The model under review builds one solid part; all positions refer to its coordinate system, in mm. A direction names the side the tool comes from. Give positions to 0.01 mm unless a question says otherwise; leave off trailing zeros. Loops run counter-clockwise (first coordinate to the right, second up) from the corner with the lowest first, then second, coordinate; pieces in that order, holes last. Notation, with made-up numbers: (79, 21.5) -> (110, 21.5) arc R15 ccw to (110, 45.5) -> close; hole circle Ø3 at (23.25, 68). An arc over 180 degrees is marked (long way). Write each question's results on one line, items separated by ' | '. Start each with the question number.
Q1. We need section D-D (x = -20). Write out the cut boundary in (y, z).
Q2. We need section A-A (y = 18.5). Write out the cut boundary in (x, z), plus the area to 3 significant figures.
Q3. We need section C-C (y = 23.5). Write out the cut boundary in (x, z), plus the area to 3 significant figures.
Q4. Insertion check: pin 1 Ø10 at (x, y) = (-17, 24.5) entering from +Z; pin 2 Ø2 at (x, z) = (3, 13.5) entering from +Y; pin 3 Ø10 at (y, z) = (15.5, 11.5) entering from +X. Each pin has a flat end and moves straight along its axis. Give the tip position at first contact, or say it passes through.
Q5. Wall thickness on L1, parallel to Z at x = 6.5, y = 15.75; L2, parallel to Y at x = -5, z = 88; L3, parallel to Y at x = -25, z = 60: over which ranges is each line inside the solid? List them lowest first. Write a range as [from, to].
Q6. Machinability: for faces 5 (the face through (20, 6, 36)), 6 (the face through (-23, 1, 44.75)), 7 (the face through (-18, 21.5, 88)), 8 (the face through (24, 20, 12)), 9 (the face through (-17, 25, 81)), which of the approach directions +Z, -Z, +X, -X, +Y, -Y give a long, thin tool a straight path to every point of the face, cutting with its end or side? Answer none if there is none.
Q7. We need section B-B (z = 26). Write out the cut boundary in (x, y).
Q8. Mouldability with a two-part tool opening along Z and no side actions: class faces 1 (the face through (-29.116, 9.513, 1.141)), 2 (the face through (0, 8, 94)), 3 (the face through (-6, 15, 93)), 4 (the face through (-7, 15.5, 36)) as released by +Z, released by -Z, zero draft, split by the parting line, or undercut.
from build123d import *

# Parameters (mm, degrees)
BOSS_EXTRUDE1_DEPTH = 94
SKETCH2_W           = 14
SKETCH2_H           = 14
CUT_EXTRUDE1_DEPTH  = 5
SKETCH3_W           = 52
SKETCH3_H           = 12
BOSS_EXTRUDE2_DEPTH = 25
SKETCH4_W           = 6
SKETCH4_H           = 48
BOSS_EXTRUDE3_DEPTH = 10
SKETCH5_W           = 13.5
SKETCH5_H           = 11
SKETCH5_W_2         = 13
SKETCH5_H_2         = 6
CUT_EXTRUDE2_DEPTH  = 10
CUT_EXTRUDE3_DEPTH  = 2
SKETCH7_W           = 19
SKETCH7_H           = 2.5
CUT_EXTRUDE4_DEPTH  = 102.056914657
SKETCH8_R           = 4
CUT_EXTRUDE5_DEPTH  = 10
BOSS_EXTRUDE5_DEPTH = 2
FILLET2_R           = 4
FILLET3_R           = 4
SKETCH10_W          = 15
SKETCH10_H          = 15
BOSS_EXTRUDE6_DEPTH = 0.5


# Some blends are built 0.0001 mm under size
with BuildPart() as part:
    # Sketch1 → Boss-Extrude1 (new body)
    with BuildSketch(Plane.XY):
        with BuildLine():
            Line((-31.5, 15.5), (-28.5, 0))
            Line((-28.5, 0), (-21, 0))
            ThreePointArc((-21, 0), (0, 1.776625594), (21, 0))
            Line((21, 0), (28.5, 0))
            Line((28.5, 0), (31.5, 15.5))
            Line((31.5, 15.5), (-31.5, 15.5))
        make_face()
    extrude(amount=BOSS_EXTRUDE1_DEPTH)

    # Sketch2 → Cut-Extrude1 (cut)
    with BuildSketch(Plane(origin=(0, 0, 0), x_dir=(-1, 0, 0), z_dir=(0, 0, -1))):
        Rectangle(SKETCH2_W, SKETCH2_H)
    extrude(amount=-CUT_EXTRUDE1_DEPTH, mode=Mode.SUBTRACT)

    # Sketch3 → Boss-Extrude2 (add)
    with BuildSketch(Plane.XY.offset(94)):
        with Locations((0, 21.5)):
            Rectangle(SKETCH3_W, SKETCH3_H)
    extrude(amount=-BOSS_EXTRUDE2_DEPTH)

    # Sketch4 → Boss-Extrude3 (add)
    with BuildSketch(Plane(origin=(0, 15.5, 0), x_dir=(1, 0, 0), z_dir=(0, 1, 0))):
        with Locations((24, -36)):
            Rectangle(SKETCH4_W, SKETCH4_H)
    extrude(amount=BOSS_EXTRUDE3_DEPTH)

    # Sketch5 → Cut-Extrude2 (cut)
    with BuildSketch(Plane.XY.offset(94)):
        with Locations((-18.25, 16)):
            Rectangle(SKETCH5_W, SKETCH5_H)
        with Locations((1, 22.5)):
            Rectangle(SKETCH5_W_2, SKETCH5_H_2)
        with Locations((19, 22.5)):
            Rectangle(SKETCH5_W_2, SKETCH5_H_2)
        with Locations((1, 13)):
            Rectangle(SKETCH5_W_2, SKETCH5_H_2)
        with Locations((19, 13)):
            Rectangle(SKETCH5_W_2, SKETCH5_H_2)
    extrude(amount=-CUT_EXTRUDE2_DEPTH, mode=Mode.SUBTRACT)

    # Sketch6 → Cut-Extrude3 (cut)
    with BuildSketch(Plane.XY.offset(94)):
        Polygon((-26, 15.5), (-26, 9.5), (-10.5, 9.5), (-10.5, 19.5), (-6, 19.5), (-6, 9.5), (8, 9.5), (8, 19.5), (12, 19.5), (12, 9.5), (26, 9.5), (26, 33.954249065), (-26, 33.954249065), align=None)
    extrude(amount=-CUT_EXTRUDE3_DEPTH, mode=Mode.SUBTRACT)

    # Sketch7 → Cut-Extrude4 (cut, through all)
    with BuildSketch(Plane.XY.offset(92)):
        with Locations((-16.5, 26.25)):
            Rectangle(SKETCH7_W, SKETCH7_H)
    extrude(amount=-CUT_EXTRUDE4_DEPTH, mode=Mode.SUBTRACT)

    # Sketch8 → Cut-Extrude5 (cut)
    with BuildSketch(Plane.XZ):
        with BuildLine():
            ThreePointArc((-21, 57.872983346), (-23.16227766, 56.449489743), (-24, 54))
            ThreePointArc((-24, 54), (-23.16227766, 51.550510257), (-21, 50.127016654))
            Line((-21, 50.127016654), (-21, 57.872983346))
        make_face()
        with BuildLine():
            ThreePointArc((-16, 54), (-17.550510257, 57.16227766), (-21, 57.872983346))
            Line((-21, 57.872983346), (-21, 50.127016654))
            ThreePointArc((-21, 50.127016654), (-17.550510257, 50.83772234), (-16, 54))
        make_face()
        with BuildLine():
            ThreePointArc((-21, 43.872983346), (-23.16227766, 42.449489743), (-24, 40))
            ThreePointArc((-24, 40), (-23.16227766, 37.550510257), (-21, 36.127016654))
            Line((-21, 36.127016654), (-21, 43.872983346))
        make_face()
        with BuildLine():
            ThreePointArc((-16, 40), (-17.550510257, 43.16227766), (-21, 43.872983346))
            Line((-21, 43.872983346), (-21, 36.127016654))
            ThreePointArc((-21, 36.127016654), (-17.550510257, 36.83772234), (-16, 40))
        make_face()
        with BuildLine():
            ThreePointArc((-16, 54), (-17.550510257, 50.83772234), (-21, 50.127016654))
            Line((-21, 50.127016654), (-21, 43.872983346))
            ThreePointArc((-21, 43.872983346), (-17.550510257, 43.16227766), (-16, 40))
            Line((-16, 40), (-16, 54))
        make_face()
        with BuildLine():
            ThreePointArc((-21, 50.127016654), (-23.16227766, 51.550510257), (-24, 54))
            Line((-24, 54), (-24, 40))
            ThreePointArc((-24, 40), (-23.16227766, 42.449489743), (-21, 43.872983346))
            Line((-21, 43.872983346), (-21, 50.127016654))
        make_face()
        with Locations((20, 54)):
            Circle(SKETCH8_R)
        with BuildLine():
            Line((24, 40), (24, 54))
            ThreePointArc((24, 54), (20, 50), (16, 54))
            Line((16, 54), (16, 40))
            ThreePointArc((16, 40), (20, 44), (24, 40))
        make_face()
        with Locations((20, 40)):
            Circle(SKETCH8_R)
    extrude(amount=-CUT_EXTRUDE5_DEPTH, mode=Mode.SUBTRACT)

    # Sketch9 → Boss-Extrude5 (add)
    with BuildSketch(Plane.XZ):
        with BuildLine():
            Line((-15, 40), (-15, 54))
            ThreePointArc((-15, 54), (-16.83772234, 57.872983346), (-21, 58.898979486))
            Line((-21, 58.898979486), (-21, 57.872983346))
            ThreePointArc((-21, 57.872983346), (-17.550510257, 57.16227766), (-16, 54))
            Line((-16, 54), (-16, 44.75))
            Line((-16, 44.75), (-18.25, 44.75))
            Line((-18.25, 44.75), (-18.25, 40))
            ThreePointArc((-18.25, 40), (-20, 38.25), (-21.75, 40))
            Line((-21.75, 40), (-21.75, 44.75))
            Line((-21.75, 44.75), (-25, 44.75))
            Line((-25, 44.75), (-25, 40))
            ThreePointArc((-25, 40), (-20, 35), (-15, 40))
        make_face()
        with BuildLine():
            Line((16, 44.75), (18.25, 44.75))
            Line((18.25, 44.75), (18.25, 40))
            ThreePointArc((18.25, 40), (20, 38.25), (21.75, 40))
            Line((21.75, 40), (21.75, 44.75))
            Line((21.75, 44.75), (25, 44.75))
            Line((25, 44.75), (25, 40))
            ThreePointArc((25, 40), (20, 35), (15, 40))
            Line((15, 40), (15, 54))
            ThreePointArc((15, 54), (16.83772234, 57.872983346), (21, 58.898979486))
            Line((21, 58.898979486), (21, 57.872983346))
            ThreePointArc((21, 57.872983346), (17.550510257, 57.16227766), (16, 54))
            Line((16, 54), (16, 44.75))
        make_face()
    extrude(amount=-BOSS_EXTRUDE5_DEPTH)

    # Fillet2
    fillet2_edges = [part.edges().sort_by_distance(p)[0] for p in [
        (-28.5, 0, 47),
        (28.5, 0, 47),
    ]]
    fillet(fillet2_edges, radius=FILLET2_R)

    # Fillet3
    fillet3_edges = [part.edges().sort_by_distance(p)[0] for p in [
        (30.313539907, 9.369956187, 0),
        (27.745510401, 0.914521876, 0),
        (23.099980206, 0, 0),
    ]]
    fillet(fillet3_edges, radius=FILLET3_R)
    fillet3_2_edges = [part.edges().sort_by_distance(p)[0] for p in [
        (-30.313539907, 9.369956187, 0),
        (-27.745510401, 0.914521876, 0),
        (-23.099980206, 0, 0),
    ]]
    fillet(fillet3_2_edges, radius=FILLET3_R)
    # the kernel refuses this fillet: 4 mm, written as the material it takes off along each edge
    with BuildSketch(Plane(origin=(29.127079814, 3.239912374, 94), x_dir=(0, 0, -1), z_dir=(0.19002190656586074, 0.9817798505902814, 0))) as fillet3_3_piece_1:
        with BuildLine():
            CenterArc((FILLET3_R, FILLET3_R), FILLET3_R, 180, 90)
            Line((0, FILLET3_R), (-FILLET3_R * 0.02, FILLET3_R))
            Line((-FILLET3_R * 0.02, FILLET3_R), (-FILLET3_R * 0.02, -FILLET3_R * 0.02))
            Line((-FILLET3_R * 0.02, -FILLET3_R * 0.02), (FILLET3_R, -FILLET3_R * 0.02))
            Line((FILLET3_R, -FILLET3_R * 0.02), (FILLET3_R, 0))
        make_face()
    extrude(amount=22.487613816, mode=Mode.SUBTRACT)
    with BuildSketch(Plane(origin=(25.199960412, 4, 94), x_dir=(0, -1, 0), z_dir=(-1, 0, 0))) as fillet3_3_piece_2:
        with BuildLine():
            CenterArc((4 - FILLET3_R, -FILLET3_R), FILLET3_R, 0, 90)
            Line((4, -FILLET3_R), (4 + FILLET3_R * 0.02, -FILLET3_R))
            Line((4 + FILLET3_R * 0.02, -FILLET3_R), (4 + FILLET3_R * 0.02, 0))
            Line((4 + FILLET3_R * 0.02, 0), (4, FILLET3_R * 0.02))
            Line((4, FILLET3_R * 0.02), (4 - FILLET3_R, FILLET3_R * 0.02))
            Line((4 - FILLET3_R, FILLET3_R * 0.02), (4 - FILLET3_R, 0))
        make_face()
    revolve(axis=Axis((25.199960412, 4, 94), (0, 0, 1)), revolution_arc=79.045937357, mode=Mode.SUBTRACT)
    with BuildSketch(Plane(origin=(11, 0, 94), x_dir=(0, 1, 0), z_dir=(1, 0, 0))) as fillet3_3_piece_3:
        with BuildLine():
            CenterArc((FILLET3_R, -FILLET3_R), FILLET3_R, 90, 90)
            Line((0, -FILLET3_R), (-FILLET3_R * 0.02, -FILLET3_R))
            Line((-FILLET3_R * 0.02, -FILLET3_R), (-FILLET3_R * 0.02, FILLET3_R * 0.02))
            Line((-FILLET3_R * 0.02, FILLET3_R * 0.02), (FILLET3_R, FILLET3_R * 0.02))
            Line((FILLET3_R, FILLET3_R * 0.02), (FILLET3_R, 0))
        make_face()
    extrude(amount=14.199960412, mode=Mode.SUBTRACT)
    fillet3_4_edges = [part.edges().sort_by_distance(p)[0] for p in [
        (-30.313539907, 9.369956187, 94),
        (-27.745510401, 0.914521876, 94),
        (-23.099980206, 0, 94),
    ]]
    fillet(fillet3_4_edges, radius=FILLET3_R - 0.0001)  # a hair under: the kernel refuses the full size

    # Sketch10 → Boss-Extrude6 (add)
    with BuildSketch(Plane(origin=(0, 15.5, 0), x_dir=(1, 0, 0), z_dir=(0, 1, 0))):
        with Locations((2, -31.5)):
            Rectangle(SKETCH10_W, SKETCH10_H)
    extrude(amount=BOSS_EXTRUDE6_DEPTH)


solid = part.part
Output:
1) outline: (0, 35) -> (0.17, 35) -> (0.17, 2.86) arc R4 ccw to (4, 0) -> (15.5, 0) -> (15.5, 69) -> (25, 69) -> (25, 92) -> (21.5, 92) -> (21.5, 84) -> (10.5, 84) -> (10.5, 92) -> (9.5, 92) -> (9.5, 94) -> (4, 94) arc R4 ccw to (0.17, 91.14) -> (0.17, 59) -> (0, 59) -> (0, 58) -> (10, 58) -> (10, 36) -> (2, 36) -> (2, 38.25) -> (0, 38.25) -> close
2) outline: (-26, 69) -> (26, 69) -> (26, 92) -> (12, 92) -> (12, 94) -> (8, 94) -> (8, 92) -> (-6, 92) -> (-6, 94) -> (-10.5, 94) -> (-10.5, 92) -> (-11.5, 92) -> (-11.5, 84) -> (-25, 84) -> (-25, 92) -> (-26, 92) -> close; (21, 12) -> (27, 12) -> (27, 60) -> (21, 60) -> close | area: 1,390 mm2
3) outline: (-26, 69) -> (26, 69) -> (26, 92) -> (25.5, 92) -> (25.5, 84) -> (12.5, 84) -> (12.5, 92) -> (7.5, 92) -> (7.5, 84) -> (-5.5, 84) -> (-5.5, 92) -> (-26, 92) -> close; (21, 12) -> (27, 12) -> (27, 60) -> (21, 60) -> close | area: 1,280 mm2
4) pin 1: z = 92 | pin 2: y = 15.5 | pin 3: x = 31.5
5) L1: [24, 39], [69, 84] | L2: [1.68, 10], [16, 19.5], [25.5, 27.5] | L3: [0, 15.5]
6) face 5: none | face 6: -Y | face 7: +Z | face 8: -Z, +X, -X, +Y | face 9: +Z, -Z, -X, +Y
7) outline: (-31.5, 15.5) -> (-29.13, 3.24) arc R4 ccw to (-25.2, 0) -> (-21, 0) arc R125 cw to (21, 0) -> (25.2, 0) arc R4 ccw to (29.13, 3.24) -> (31.5, 15.5) -> (27, 15.5) -> (27, 25.5) -> (21, 25.5) -> (21, 15.5) -> (9.5, 15.5) -> (9.5, 16) -> (-5.5, 16) -> (-5.5, 15.5) -> close
8) face 1: released by -Z | face 2: released by +Z | face 3: zero draft | face 4: undercut
